from build123d import *

# Parameters (mm, degrees)
SKETCH005_R      = 4.125
EXTRUDE007_DEPTH = 4
EXTRUDE004_DEPTH = 44


with BuildPart() as extrude007:
    # Sketch005 → Extrude007 (new body)
    with BuildSketch(Plane.XZ):
        Polygon((24, 74), (98, 0), (98, -30), (94, -30), (53, -30), (49, -30), (45, -30), (4, -30), (0, -30), (-4, -30), (-45, -30), (-49, -30), (-53, -30), (-94, -30), (-98, -30), (-98, 0), (-24, 74), (-20, 74), (20, 74), align=None)
        with Locations((-49, 4.125)):
            Circle(SKETCH005_R, mode=Mode.SUBTRACT)
        with Locations((49, 4.125)):
            Circle(SKETCH005_R, mode=Mode.SUBTRACT)
        with Locations((0, 41.339394)):
            Circle(SKETCH005_R, mode=Mode.SUBTRACT)
    extrude(amount=EXTRUDE007_DEPTH)


with BuildPart() as stage_3_paths:
    # Sketch → Extrude004 (new body)
    with BuildSketch(Plane.XZ):
        Polygon((-20, 74), (-94, 0), (-94, -30), (-96, -28.845299), (-98, -30), (-98, 0), (-24, 74), (-22, 75.154701), align=None)
        Polygon((24, 74), (98, 0), (98, -30), (96, -28.845299), (94, -30), (94, 0), (20, 74), (22, 75.154701), align=None)
        Polygon((4, 37.339394), (-4, 37.339394), (-13.145979, 28.193415), (-13.145979, 24.193415), (-4, 33.339394), (-4, 0), (-4, -30), (-2, -28.845299), (0, -30), (2, -28.845299), (4, -30), (4, 0), (4, 33.339394), (13.145979, 24.193415), (13.145979, 28.193415), align=None)
        Polygon((-53, 0), (-45, 0), (-45, -30), (-47, -28.845299), (-49, -30), (-51, -28.845299), (-53, -30), align=None)
        Polygon((45, 0), (53, 0), (53, -30), (51, -28.845299), (49, -30), (47, -28.845299), (45, -30), align=None)
    extrude(amount=EXTRUDE004_DEPTH)


with BuildPart() as stage_3_paths_1:
    # Extrude004 placement: moved
    add(stage_3_paths.part.moved(Location((0, -4, 0))))

    # Fusion005: union Extrude007
    add(extrude007.part)


solid = stage_3_paths_1.part
Read the model definition and answer for the solid it produces. Units are mm, in the model's axes. A direction names the side the tool comes from. Coordinates: 2 decimals unless noted, no trailing zeros. Loops run counter-clockwise (first coordinate to the right, second up) from the corner with the lowest first, then second, coordinate; pieces in that order, holes last. Notation, with made-up numbers: (51, 84) - (65, 84) arc R16 ccw to (65, 95) - close; hole circle Ø7 at (60, 7). An arc over 180 degrees is marked (long way). Answer in a Markdown table with one row per item.
Q1. Find section A-A on z = -15.5. Write down the section's boundary in (x, y), plus the area to 3 significant figures.
Here are the results:
| item | result |
|---|---|
| outline | (-98, -48) - (-94, -48) - (-94, -4) - (-53, -4) - (-53, -48) - (-45, -48) - (-45, -4) - (-4, -4) - (-4, -48) - (4, -48) - (4, -4) - (45, -4) - (45, -48) - (53, -48) - (53, -4) - (94, -4) - (94, -48) - (98, -48) - (98, 0) - (-98, 0) - close |
| area | 2,190 mm^2 |
Q2. Find section C-C on y = -12.5. Count the separate pieces of the cut face and the enclosed holes in it, plus the area to 3 significant figures.
Here are the results:
| item | result |
|---|---|
| separate pieces | 5 |
| enclosed holes | 0 |
| area | 1,910 mm^2 |
Q3. The mould has two halves that part along Z. Classify faces 6 (the flat face through (45, -26, -15)), 7 (the flat face through (49, -26, 0)), 8 (the flat face through (0, -2, 74)): pulls with the +Z half, pulls with the -Z half, needs draft (parallel to the pull), parting line crosses it, or undercut.
Here are the results:
| item | result |
|---|---|
| face 6 | needs draft |
| face 7 | undercut |
| face 8 | pulls with the +Z half |
Q4. Straight lines are drawn through the part: line 1 along X through (y, z) = (-34, -9); line 2 along X through (y, z) = (-38, 16); line 3 along X through (y, z) = (-29, 31). For each, find the intervals that lie inside material, in ascending order. Write a range as [from, to].
Here are the results:
| item | result |
|---|---|
| line 1 | x = [-98, -94], [-53, -45], [-4, 4], [45, 53], [94, 98] |
| line 2 | x = [-82, -78], [-4, 4], [78, 82] |
| line 3 | x = [-67, -63], [-10.34, -6.34], [-4, 4], [6.34, 10.34], [63, 67] |
Q5. For faces 1 (the cylindrical face through (-53.12, -1.97, 4.31)), 2 (the flat face through (-49, -48, -15)), 3 (the flat face through (-8.51, -25.69, 32.83)), 4 (the flat face through (13.146, -26, 26)), 5 (the flat face through (-45, -26, -15)), determine the directions among +Z, -Z, +X, -X, +Y, -Y from which every point of the face is accessible in a straight line to the end or side of a thin tool.
Here are the results:
| item | result |
|---|---|
| face 1 | +Y, -Y |
| face 2 | +Z, -Z, +X, -X, -Y |
| face 3 | +Z, -Y |
| face 4 | +Z, -Z, -Y |
| face 5 | -Z, -Y |
Q6. Find section D-D on z = 49. Write down the section's boundary in (x, y).
Here are the results:
| item | result |
|---|---|
| outline | (-49, -48) - (-45, -48) - (-45, -4) - (45, -4) - (45, -48) - (49, -48) - (49, 0) - (-49, 0) - close |
Q7. Given P1, Ø1.5, axis at x = 67, z = 9.5, coming from the -Y side; P2, Ø1.3, axis at x = 22.5, z = 75, coming from the +Y side; P3, Ø9, axis at x = -0.5, y = -15.5, coming from the +Z side, each flat-ended and moving along its own axis, determine where each tip first touches the part or whether it passes through.
Here are the results:
| item | result |
|---|---|
| P1 | stops at y = -4 |
| P2 | stops at y = -4 |
| P3 | stops at z = 37.34 |
Q8. Find section B-B on x = 59. Write down the section's boundary in (y, z).
Here are the results:
| item | result |
|---|---|
| outline | (-48, 35) - (-4, 35) - (-4, -30) - (0, -30) - (0, 39) - (-48, 39) - close |
